```python
from build123d import *

# Parameters (mm, degrees)
PAD_DEPTH       = 70
SKETCH001_R     = 2.75
SKETCH001_R_2   = 4
POCKET_DEPTH    = 25.251
SKETCH002_R     = 4.75
POCKET001_DEPTH = 20.251
FILLET_R        = 3


with BuildPart() as part:
    # Sketch → Pad (new body)
    with BuildSketch(Plane.XY):
        with BuildLine():
            ThreePointArc((14.716063, 0), (0, 13.75), (-14.716063, 0))
            Line((-26.230945, 0), (-14.716063, 0))
            ThreePointArc((26.230945, 0), (0, 25.25), (-26.230945, 0))
            Line((14.716063, 0), (26.230945, 0))
        make_face()
    extrude(amount=PAD_DEPTH)

    # Sketch001 (on Face2 of Pad) → Pocket (cut, through all)
    with BuildSketch(Plane.XZ):
        with Locations((-19.25, 17.5)):
            Circle(SKETCH001_R)
        with Locations((19.25, 17.5)):
            Circle(SKETCH001_R)
        with Locations((0, 15)):
            Circle(SKETCH001_R_2)
        with Locations((19.25, 52.5)):
            Circle(SKETCH001_R)
        with Locations((-19.25, 52.5)):
            Circle(SKETCH001_R)
    extrude(amount=-POCKET_DEPTH, mode=Mode.SUBTRACT)

    # Sketch002 (on DatumPlane) → Pocket001 (cut, through all)
    with BuildSketch(Plane.XZ.offset(-5)):
        with Locations((-19.25, 17.5)):
            Circle(SKETCH002_R)
        with Locations((-19.25, 52.5)):
            Circle(SKETCH002_R)
        Polygon((19.25, 12.592523), (23.5, 15.046261), (23.5, 19.953739), (19.25, 22.407477), (15, 19.953739), (15, 15.046261), align=None)
        Polygon((19.25, 47.592523), (23.5, 50.046261), (23.5, 54.953739), (19.25, 57.407477), (15, 54.953739), (15, 50.046261), align=None)
    extrude(amount=-POCKET001_DEPTH, mode=Mode.SUBTRACT)

    # Fillet
    fillet_edges = [part.edges().sort_by_distance(p)[0] for p in [
        (0, 25.25, 70),
    ]]
    fillet(fillet_edges, radius=FILLET_R)


solid = part.part
```
CAD build for the part. Positions are in the model's coordinates, mm. A direction names the side the tool comes from. Coordinates: 2 decimals unless noted, no trailing zeros. Write each loop counter-clockwise with the first axis right and the second up, starting at its lowest first coordinate (ties: lowest second). Pieces come first, ordered by that corner, then holes.
(1) Two-plate mould, pull along X, no slides. Class faces 3 (the face through (17.095, 12.662, 13.837)), 4 (the face through (-19.608, 2.465, 55.227)), 5 (the face through (0.563, 25.244, 33.031)), 6 (the face through (0, 16, 0)): +X half, -X half, draft (parallel to the pull), parting line (faces both ways), or undercut.
(2) Cut at B-B, the plane y = 3.5. Count the separate pieces of the cut face and the enclosed holes in it, and give its area (3 significant figures).
(3) Cut at A-A, the plane x = 0. List the corners of the cut face in (y, z).
(4) 3-axis set-ups, long thin cutter, end or side, ignore diameter. For faces 1 (the face through (18.892, 2.465, 20.227)), 2 (the face through (23.5, 8, 52)): which of +Z, -Z, +X, -X, +Y, -Y reach the whole face in a straight line?
(5) Cut at C-C, the plane z = 40. List the corners of the cut face in (x, y), and give its area (3 significant figures).
(6) Drill centre lines: probe 1 along Z at (x, y) = (19.25, 1.4); probe 2 along Y at (x, z) = (22.5, 54); probe 3 along X at (y, z) = (15, 52.5). Where is each one in solid material? Low to high.
(7) Flat gauge pins, fed straight in: pin 1 (9 mm diameter, centred on x = 19.25, z = 17.5, fed in from -Y); pin 2 (6 mm diameter, centred on y = 9.5, z = 30, fed in from -X); pin 3 (7.5 mm diameter, centred on x = -18.5, z = 52.5, fed in from +Y); pin 4 (6 mm diameter, centred on x = -6, z = 9.5, fed in from +Y). Where does each tip first touch, or does it go through?
Geometry says:
1. face 3: undercut
1. face 4: undercut
1. face 5: parting line
1. face 6: draft
2. separate pieces: 2
2. enclosed holes: 4
2. area: 1,560 mm2
3. outline: (13.75, 0) - (25.25, 0) - (25.25, 11) - (13.75, 11) - close; (13.75, 19) - (25.25, 19) - (25.25, 67) arc R3 ccw to (22.25, 70) - (13.75, 70) - close
4. face 1: +Y, -Y
4. face 2: +Y
5. outline: (-26.23, 0) - (-14.72, 0) arc R14.75 cw to (14.72, 0) - (26.23, 0) arc R26.25 ccw to start
5. area: 718 mm2
6. probe 1: z = 0 to 14.75, 20.25 to 49.75, 55.25 to 70
6. probe 2: y = 0 to 5
6. probe 3: x = -14.5 to 15
7. pin 1: stops at y = 0
7. pin 2: stops at x = -25.16
7. pin 3: stops at y = 5
7. pin 4: stops at y = 25.08
